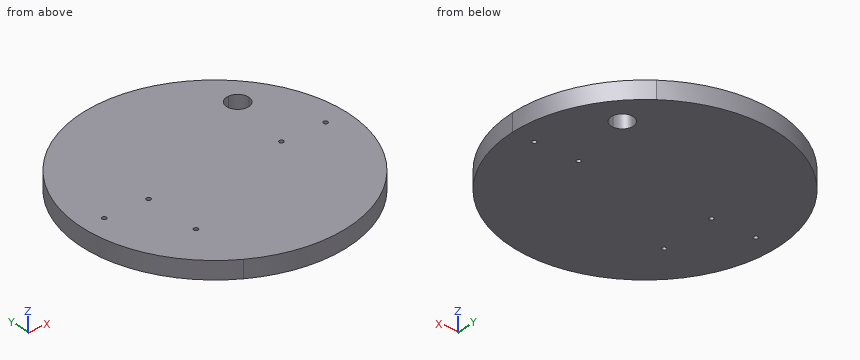
```python
from build123d import *

# Parameters (mm, degrees)
F0_R     = 1
F1_DEPTH = 8


with BuildPart() as f1:
    # F0 (on Top) → F1 (new body)
    with BuildSketch(Plane.XY):
        with BuildLine():
            ThreePointArc((-30, -51.961524), (30, -51.961524), (60, 0))
            ThreePointArc((60, 0), (53.385391, 27.386128), (35, 48.733972))
            ThreePointArc((35, 48.733972), (-50.409778, 32.540041), (-30, -51.961524))
        make_face()
        with BuildLine():
            ThreePointArc((-29, -25.980762), (-29.292893, -26.687869), (-30, -26.980762))
            ThreePointArc((-30, -26.980762), (-31, -25.980762), (-30, -24.980762))
            ThreePointArc((-30, -24.980762), (-29.292893, -25.273655), (-29, -25.980762))
        make_face(mode=Mode.SUBTRACT)
        with Locations((-50, 0)):
            Circle(F0_R, mode=Mode.SUBTRACT)
        with BuildLine():
            ThreePointArc((-29, 0), (-29.292893, -0.707107), (-30, -1))
            ThreePointArc((-30, -1), (-30.707107, 0.707107), (-29, 0))
        make_face(mode=Mode.SUBTRACT)
        with Locations((30, 0)):
            Circle(F0_R, mode=Mode.SUBTRACT)
        with Locations((50, 0)):
            Circle(F0_R, mode=Mode.SUBTRACT)
        with BuildLine():
            ThreePointArc((35, 25), (30, 30), (35, 35))
            ThreePointArc((35, 35), (38.535534, 33.535534), (40, 30))
            ThreePointArc((40, 30), (38.535534, 26.464466), (35, 25))
        make_face(mode=Mode.SUBTRACT)
    extrude(amount=F1_DEPTH)


solid = f1.part
```
CAD build for the part. Positions are in the model's coordinates, mm. Coordinates: 2 decimals unless noted, no trailing zeros. Order: outer loops, then holes, each group sorted by start corner. A loop starts at its lowest first (then second) coordinate and runs counter-clockwise, first axis right, second up.
(1) Saw through at A-A, the plane z = 3.75. Write the cut outline in (x, y).
Solution:
outline: (35, 48.73) arc R60 ccw (long way) to (60, 0) arc R60 ccw to start; hole circle Ø2 at (-50, 0); hole circle Ø2 at (-30, 0); hole (-30, -24.98) arc R1 ccw (long way) to (-29, -25.98) arc R1 ccw to start; hole circle Ø2 at (30, 0); hole circle Ø10 at (35, 30); hole circle Ø2 at (50, 0)
(2) Drill centre lines: L1, parallel to Y at x = -30, z = 4.5; L2, parallel to Y at x = -1, z = 2.5; L3, parallel to X at y = 21.5, z = 5.25. Where is each one in solid material? Low to high.
Solution:
L1: y = -51.96 to -26.98, -24.98 to -1, 1 to 51.96
L2: y = -59.99 to 59.99
L3: x = -56.02 to 56.02
(3) Pin check, flat tips, straight feed: pin 1 Ø2.5 at (x, y) = (30, 0) entering from +Z; pin 2 Ø1 at (x, z) = (7.5, 4.5) entering from +Y; pin 3 Ø4 at (y, z) = (-33.5, 6.5) entering from +X; pin 4 Ø1.5 at (x, z) = (13.5, 2) entering from +Y. Stop position of each tip, or through.
Solution:
pin 1: stops at z = 8
pin 2: stops at y = 59.59
pin 3: stops at x = 51.07
pin 4: stops at y = 58.63
(4) Saw through at B-B, the plane y = -19. Write the cut outline in (x, z).
Solution:
outline: (-56.91, 0) - (56.91, 0) - (56.91, 8) - (-56.91, 8) - close
(5) Saw through at C-C, the plane x = 23. Write the cut outline in (y, z).
Solution:
outline: (-55.42, 0) - (55.42, 0) - (55.42, 8) - (-55.42, 8) - close
